```python
from build123d import *

# Parameters (mm, degrees)
F0_W     = 127
F0_H     = 76.2
F1_DEPTH = 12.7
F2_R     = 6.35
F3_DEPTH = 12.701
F4_W     = 12.7
F4_H     = 50.8
F6_W     = 15.515666
F6_H     = 6.35
F8_SIZE  = 2.54
F9_R     = 2.54


with BuildPart() as f1:
    # F0 (on Top) → F1 (new body)
    with BuildSketch(Plane.XY):
        Rectangle(F0_W, F0_H)
    extrude(amount=F1_DEPTH)

    # F2 (on face) → F3 (cut, through all)
    with BuildSketch(Plane.XY.offset(12.7)):
        with Locations((-50.8, -25.4)):
            Circle(F2_R)
        with Locations((50.8, 25.4)):
            Circle(F2_R)
        with Locations((50.8, -25.4)):
            Circle(F2_R)
        with Locations((-50.8, 25.4)):
            Circle(F2_R)
    extrude(amount=-F3_DEPTH, mode=Mode.SUBTRACT)

    # F4 (on Front) → F5 (revolve)
    with BuildSketch(Plane.XZ):
        with Locations((6.35, 38.1)):
            Rectangle(F4_W, F4_H)
    revolve(axis=Axis((0, 0, 38.1), (0, 0, 1)))

    # F6 (on Front) → F7 (revolve, cut)
    with BuildSketch(Plane.XZ):
        with Locations((17.917833, 41.275)):
            Rectangle(F6_W, F6_H)
    revolve(axis=Axis((0, 0, 12.7), (0, 0, 1)), mode=Mode.SUBTRACT)

    # F8
    f8_edges = [f1.edges().sort_by_distance(p)[0] for p in [
        (0, -38.1, 12.7),
        (63.5, 0, 12.7),
        (0, 38.1, 12.7),
        (-63.5, 0, 12.7),
    ]]
    chamfer(f8_edges, length=F8_SIZE)

    # F9
    f9_edges = [f1.edges().sort_by_distance(p)[0] for p in [
        (-12.7, 0, 12.7),
        (-12.7, 0, 63.5),
    ]]
    fillet(f9_edges, radius=F9_R)


solid = f1.part
```
CAD build for the part. Positions are in the model's coordinates, mm. A direction names the side the tool comes from. Round coordinates to 2 decimals unless told otherwise and drop trailing zeros. Order: outer loops, then holes, each group sorted by start corner. A loop starts at its lowest first (then second) coordinate and runs counter-clockwise, first axis right, second up. Notation, with made-up numbers: (-0.5, 40.5) -> (36.5, 40.5) arc R15 ccw to (36.5, 48.5) -> close; hole circle Ø8 at (39, 77). An arc over 180 degrees is marked (long way). Write item = value, one per line.
(1) Drill centre lines: L1, parallel to X at y = 25, z = 9; L2, parallel to Y at x = 50.8, z = 7.5; L3, parallel to Y at x = 50.8, z = 10.25. Where is each one in solid material? Low to high.
Answers follow:
L1 = -63.5 to -57.14, -44.46 to 44.46, 57.14 to 63.5
L2 = -38.1 to -31.75, -19.05 to 19.05, 31.75 to 38.1
L3 = -38.01 to -31.75, -19.05 to 19.05, 31.75 to 38.01
(2) 3-axis set-ups, long thin cutter, end or side, ignore diameter. For faces 1 (the cylindrical face through (-2.75, -12.4, 52.82)), 2 (the flat face through (0, 0, 63.5)), 3 (the flat face through (6, 9, 44.45)): which of +Z, -Z, +X, -X, +Y, -Y reach the whole face in a straight line?
Answers follow:
face_1 = +Z
face_2 = +Z, +X, -X, +Y, -Y
face_3 = none
(3) Cut at C-C (x = 0). Write the cut outline in (y, z).
Answers follow:
outline = (-38.1, 0) -> (38.1, 0) -> (38.1, 10.16) -> (35.56, 12.7) -> (15.24, 12.7) arc R2.54 cw to (12.7, 15.24) -> (12.7, 38.1) -> (10.16, 38.1) -> (10.16, 44.45) -> (12.7, 44.45) -> (12.7, 60.96) arc R2.54 ccw to (10.16, 63.5) -> (-10.16, 63.5) arc R2.54 ccw to (-12.7, 60.96) -> (-12.7, 44.45) -> (-10.16, 44.45) -> (-10.16, 38.1) -> (-12.7, 38.1) -> (-12.7, 15.24) arc R2.54 cw to (-15.24, 12.7) -> (-35.56, 12.7) -> (-38.1, 10.16) -> close
(4) Flat gauge pins, fed straight in: P1, Ø7.5, axis at x = 50.8, y = 25.4, coming from the -Z side; P2, Ø6, axis at x = 35.5, y = -6, coming from the +Z side; P3, Ø10, axis at y = -3, z = 34.5, coming from the -X side; P4, Ø6, axis at x = -6, z = 27.5, coming from the -Y side. Where does each tip first touch, or does it go through?
Answers follow:
P1 = through
P2 = 12.7
P3 = -12.7
P4 = -12.34
(5) Cut at D-D (y = 0). Write the cut outline in (x, z), plus the area to 3 significant figures.
Answers follow:
outline = (-63.5, 0) -> (63.5, 0) -> (63.5, 10.16) -> (60.96, 12.7) -> (15.24, 12.7) arc R2.54 cw to (12.7, 15.24) -> (12.7, 38.1) -> (10.16, 38.1) -> (10.16, 44.45) -> (12.7, 44.45) -> (12.7, 60.96) arc R2.54 ccw to (10.16, 63.5) -> (-10.16, 63.5) arc R2.54 ccw to (-12.7, 60.96) -> (-12.7, 44.45) -> (-10.16, 44.45) -> (-10.16, 38.1) -> (-12.7, 38.1) -> (-12.7, 15.24) arc R2.54 cw to (-15.24, 12.7) -> (-60.96, 12.7) -> (-63.5, 10.16) -> close
area = 2,860 mm²
(6) Cut at B-B (x = 50.8). Write the cut outline in (y, z), plus the area to 3 significant figures.
Answers follow:
outline = (-38.1, 0) -> (-31.75, 0) -> (-31.75, 12.7) -> (-35.56, 12.7) -> (-38.1, 10.16) -> close; (-19.05, 0) -> (19.05, 0) -> (19.05, 12.7) -> (-19.05, 12.7) -> close; (31.75, 0) -> (38.1, 0) -> (38.1, 10.16) -> (35.56, 12.7) -> (31.75, 12.7) -> close
area = 639 mm²
(7) Cut at A-A (y = 25.4). Write the cut outline in (x, z).
Answers follow:
outline = (-63.5, 0) -> (-57.15, 0) -> (-57.15, 12.7) -> (-60.96, 12.7) -> (-63.5, 10.16) -> close; (-44.45, 0) -> (44.45, 0) -> (44.45, 12.7) -> (-44.45, 12.7) -> close; (57.15, 0) -> (63.5, 0) -> (63.5, 10.16) -> (60.96, 12.7) -> (57.15, 12.7) -> close
(8) Pull direction X, two halves, no side cores. Call faces 4 (the flat face through (63.5, -1, 5)), 5 (the flat face through (-63.5, -1, 5)), 6 (the cylindrical face through (56.666, -27.832, 6.439)): +X half, -X half, draft (parallel to the pull), parting line (faces both ways), or undercut.
Answers follow:
face_4 = +X half
face_5 = -X half
face_6 = undercut
